The drawing under review shows one solid part. Ordinate dimensions are in mm from its lowest x, y, z. Give positions to 0.01 mm unless a question says otherwise; leave off trailing zeros. Order: outer loops, then holes, each group sorted by start corner. A loop starts at its lowest first (then second) coordinate and runs counter-clockwise, first axis right, second up. Notation, with made-up numbers: (-14.75, 19) -> (0.25, 19) arc R19 ccw to (0.25, 34) -> close; hole circle Ø8 at (88.25, 29). An arc over 180 degrees is marked (long way). One line per item, written item: value. Start each with the question number.
1) Consider section A-A (z = 6.75). State the section outline as (x, y) points.
2) Consider section C-C (y = 18). State the section outline as (x, z) points.
3) Consider section B-B (x = 36). State the section outline as (y, z) points.
4) Consider section D-D (y = 7). State the section outline as (x, z) points.
5) The part is to be moulded in two halves that separate along Y. For the marked faces 1 and 2, say which applies: released by +Y, released by -Y, zero draft, split by the parting line, or undercut.
6) Wall thickness on line 1 along Y through (x, z) = (5, 3.75); line 2 along Y through (x, z) = (4.5, 0.5); line 3 along Y through (x, z) = (35.5, 1.5): over which ranges is each line inside the solid? List them lowest first. Write a range as from..to.
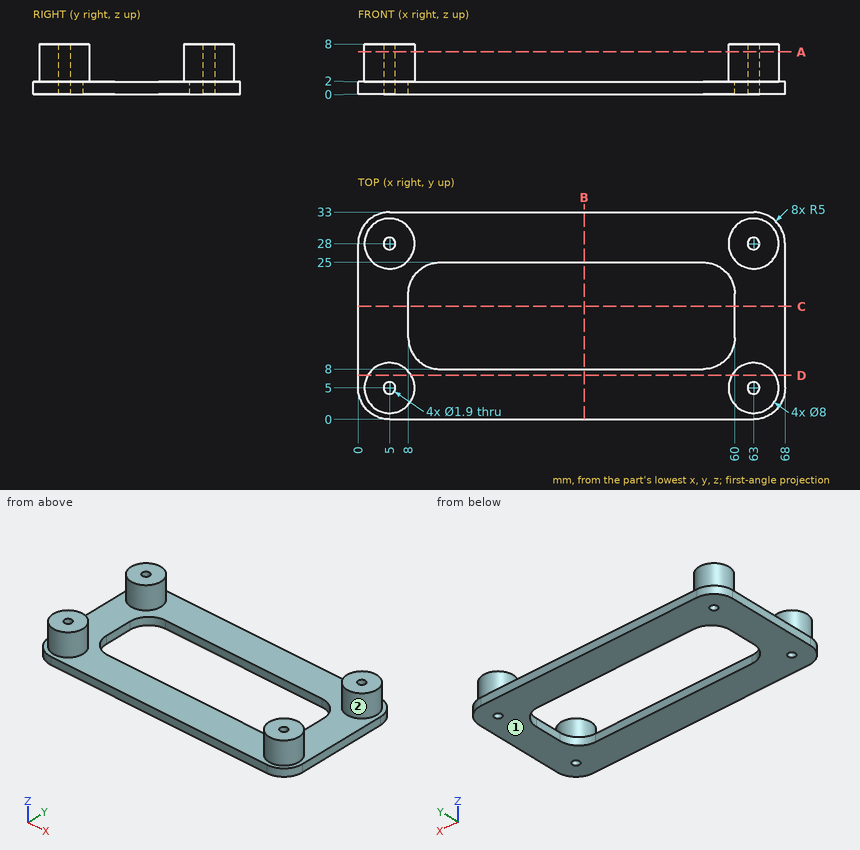
Checked values:
1. outline: circle Ø8 at (5, 5); circle Ø8 at (5, 28); circle Ø8 at (63, 5); circle Ø8 at (63, 28); hole circle Ø1.9 at (5, 5); hole circle Ø1.9 at (5, 28); hole circle Ø1.9 at (63, 5); hole circle Ø1.9 at (63, 28)
2. outline: (0, 0) -> (8, 0) -> (8, 2) -> (0, 2) -> close; (60, 0) -> (68, 0) -> (68, 2) -> (60, 2) -> close
3. outline: (0, 0) -> (8, 0) -> (8, 2) -> (0, 2) -> close; (25, 0) -> (33, 0) -> (33, 2) -> (25, 2) -> close
4. outline: (0, 0) -> (68, 0) -> (68, 2) -> (66.46, 2) -> (66.46, 8) -> (59.54, 8) -> (59.54, 2) -> (8.46, 2) -> (8.46, 8) -> (1.54, 8) -> (1.54, 2) -> (0, 2) -> close
5. face 1: zero draft
5. face 2: undercut
6. line 1: y = 1..4.05, 5.95..9, 24..27.05, 28.95..32
6. line 2: y = 0.03..4.19, 5.81..27.19, 28.81..32.97
6. line 3: y = 0..8, 25..33
